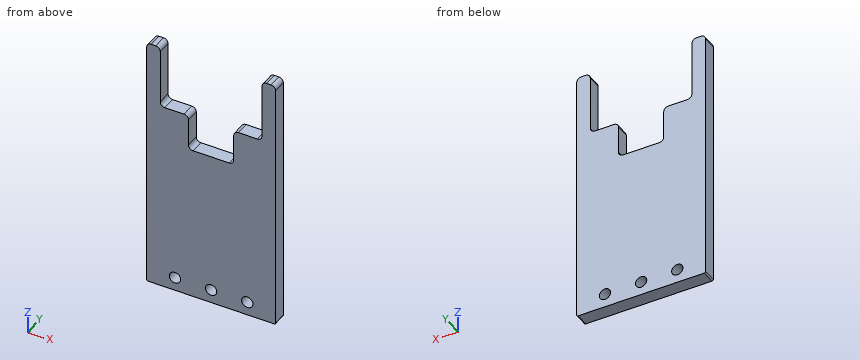
```python
from build123d import *

# Parameters (mm, degrees)
SKETCH1_W             = 28.5
SKETCH1_H             = 42.75
BOSS_EXTRUDE1_DEPTH   = 3
M3X0_5_TAPPED_HOLE1_D = 2.5
SKETCH6_W             = 3
SKETCH6_H             = 14
BOSS_EXTRUDE2_DEPTH   = 3
SKETCH7_W             = 10
SKETCH7_H             = 8
CUT_EXTRUDE1_DEPTH    = 52.466615393
FILLET1_R             = 1
FILLET2_R             = 0.3


with BuildPart() as part:
    # Sketch1 → Boss-Extrude1 (new body)
    with BuildSketch(Plane(origin=(0, 0, 0), x_dir=(1, 0, 0), z_dir=(0, 1, 0))):
        with Locations((14.25, 21.375)):
            Rectangle(SKETCH1_W, SKETCH1_H)
    extrude(amount=BOSS_EXTRUDE1_DEPTH)

    # M3x0.5 Tapped Hole1 (through all)
    with Locations(Plane(origin=(0, 0, 0), x_dir=(-1, 0, 0), z_dir=(0, -1, 0))):
        with Locations((-22.25, 39.75), (-14.25, 39.75), (-6.25, 39.75)):
            Hole(M3X0_5_TAPPED_HOLE1_D / 2)

    # Sketch6 → Boss-Extrude2 (add)
    with BuildSketch(Plane(origin=(0, 3, 0), x_dir=(1, 0, 0), z_dir=(0, 1, 0))):
        with Locations((1.5, -7)):
            Rectangle(SKETCH6_W, SKETCH6_H)
        with Locations((27, -7)):
            Rectangle(SKETCH6_W, SKETCH6_H)
    extrude(amount=-BOSS_EXTRUDE2_DEPTH)

    # Sketch7 → Cut-Extrude1 (cut, through all)
    with BuildSketch(Plane(origin=(0, 3, 0), x_dir=(1, 0, 0), z_dir=(0, 1, 0))):
        with Locations((14.25, 4)):
            Rectangle(SKETCH7_W, SKETCH7_H)
    extrude(amount=-CUT_EXTRUDE1_DEPTH, mode=Mode.SUBTRACT)

    # Fillet1
    fillet1_edges = [part.edges().sort_by_distance(p)[0] for p in [
        (3, 1.5, 0),
        (3, 1.5, 14),
        (0, 1.5, 14),
        (25.5, 1.5, 14),
        (25.5, 1.5, 0),
        (28.5, 1.5, 14),
        (19.25, 1.5, -8),
        (19.25, 1.5, 0),
        (9.25, 1.5, 0),
        (9.25, 1.5, -8),
    ]]
    fillet(fillet1_edges, radius=FILLET1_R)

    # Fillet2
    fillet2_edges = [part.edges().sort_by_distance(p)[0] for p in [
        (0, 1.5, -42.75),
        (28.5, 1.5, -42.75),
    ]]
    fillet(fillet2_edges, radius=FILLET2_R)


solid = part.part
```
The model under review builds one solid part; all positions refer to its coordinate system, in mm. Give positions to 0.01 mm unless a question says otherwise; leave off trailing zeros. Write each loop counter-clockwise with the first axis right and the second up, starting at its lowest first coordinate (ties: lowest second). Pieces come first, ordered by that corner, then holes. Notation, with made-up numbers: M 11.25,-1 L 47.25,-1 A13 ccw 47.25,18 Z; hole C 31,20.5 d3. An arc over 180 degrees is marked long. Write item = value, one per line. Start each with the question number.
Q1. For line 1 (X direction, y = 2, z = -39.75); line 2 (X direction, y = 2.15, z = -2); line 3 (Z direction, x = 22.25, y = 1.2), list the stretches that pass through material, from the lowest coordinate up.
Q2. We need section A-A (z = -2.5). State the section outline as (x, y) points, plus the area to 3 significant figures.
Q3. We need section C-C (y = 1.25). State the section outline as (x, z) points.
Q4. We need section B-B (x = 22.25). State the section outline as (y, z) points.
Q5. Clearance check with a flat-ended pin moving along its axis: pin 1 (0.9 mm diameter, centred on x = 13, y = 1, fed in from +Z). State where the tip first meets the part, or that it passes through.
Q6. We need section D-D (z = -39.75). State the section outline as (x, y) points.
Result set:
q1.line_1 = 0 to 5, 7.5 to 13, 15.5 to 21, 23.5 to 28.5
q1.line_2 = 0 to 9.25, 19.25 to 28.5
q1.line_3 = -42.75 to -41, -38.5 to 0
q2.outline = M 0,0 L 9.25,0 L 9.25,3 L 0,3 Z; M 19.25,0 L 28.5,0 L 28.5,3 L 19.25,3 Z
q2.area = 55.5 mm2
q3.outline = M 0,-42.45 A0.3 ccw 0.3,-42.75 L 28.2,-42.75 A0.3 ccw 28.5,-42.45 L 28.5,13 A1 ccw 27.5,14 L 26.5,14 A1 ccw 25.5,13 L 25.5,1 A1 cw 24.5,0 L 20.25,0 A1 ccw 19.25,-1 L 19.25,-7 A1 cw 18.25,-8 L 10.25,-8 A1 cw 9.25,-7 L 9.25,-1 A1 ccw 8.25,0 L 4,0 A1 cw 3,1 L 3,13 A1 ccw 2,14 L 1,14 A1 ccw 0,13 Z; hole C 6.25,-39.75 d2.5; hole C 14.25,-39.75 d2.5; hole C 22.25,-39.75 d2.5
q4.outline = M 0,-42.75 L 3,-42.75 L 3,-41 L 0,-41 Z; M 0,-38.5 L 3,-38.5 L 3,0 L 0,0 Z
q5.pin_1 = -8
q6.outline = M 0,0 L 5,0 L 5,3 L 0,3 Z; M 7.5,0 L 13,0 L 13,3 L 7.5,3 Z; M 15.5,0 L 21,0 L 21,3 L 15.5,3 Z; M 23.5,0 L 28.5,0 L 28.5,3 L 23.5,3 Z
